from build123d import *

# Parameters (mm, degrees)
SKETCH1_W               = 100
SKETCH1_H               = 45
BOSS_EXTRUDE1_DEPTH     = 3
BOSS_EXTRUDE2_DEPTH     = 15
SKETCH4_R               = 1.5
CUT_EXTRUDE1_DEPTH      = 79
SKETCH5_R               = 1.5
CUT_EXTRUDE2_DEPTH      = 25
FILLET1_R               = 2
SKETCH6_W               = 3
SKETCH6_H               = 45
BOSS_EXTRUDE3_DEPTH     = 20
FILLET2_R               = 17
SKETCH7_R               = 1.75
CUT_EXTRUDE3_DEPTH      = 73.5
CIRPATTERN1_COUNT       = 5
CIRPATTERN1_ANGLE       = 80
MIRROR1_COPY_1_SKETCH_R = 1.75
MIRROR1_COPY_1_DEPTH    = 73.5
MIRROR1_COPY_2_SKETCH_R = 1.75
MIRROR1_COPY_2_DEPTH    = 73.5
MIRROR1_COPY_3_SKETCH_R = 1.75
MIRROR1_COPY_3_DEPTH    = 73.5
MIRROR1_COPY_4_SKETCH_R = 1.75
MIRROR1_COPY_4_DEPTH    = 73.5
SKETCH8_R               = 1.75
CUT_EXTRUDE4_DEPTH      = 24
LPATTERN1_COUNT         = 4
LPATTERN1_PITCH         = 5
MIRROR2_COPY_1_SKETCH_R = 1.75
MIRROR2_COPY_1_DEPTH    = 24
MIRROR2_COPY_2_SKETCH_R = 1.75
MIRROR2_COPY_2_DEPTH    = 24
MIRROR2_COPY_3_SKETCH_R = 1.75
MIRROR2_COPY_3_DEPTH    = 24


with BuildPart() as part:
    # Sketch1 → Boss-Extrude1 (new body)
    with BuildSketch(Plane(origin=(0, 0, 0), x_dir=(1, 0, 0), z_dir=(0, 1, 0))):
        Rectangle(SKETCH1_W, SKETCH1_H)
    extrude(amount=BOSS_EXTRUDE1_DEPTH)

    # Sketch2 → Boss-Extrude2 (add)
    with BuildSketch(Plane(origin=(0, 3, 0), x_dir=(1, 0, 0), z_dir=(0, 1, 0))):
        Polygon((-25, 22.5), (-28, 22.5), (-28, -22.5), (-25, -22.5), (-25, -1.5), (25, -1.5), (25, -22.5), (28, -22.5), (28, 22.5), (25, 22.5), (25, 1.5), (-25, 1.5), align=None)
    extrude(amount=BOSS_EXTRUDE2_DEPTH)

    # Sketch4 → Cut-Extrude1 (cut, through all)
    with BuildSketch(Plane.ZY.offset(28)):
        with Locations((-18.5, 9.88505799)):
            Circle(SKETCH4_R)
        with Locations((18.5, 9.88505799)):
            Circle(SKETCH4_R)
    extrude(amount=-CUT_EXTRUDE1_DEPTH, mode=Mode.SUBTRACT)

    # Sketch5 → Cut-Extrude2 (cut, through all)
    with BuildSketch(Plane.XY.offset(1.5)):
        with Locations((-18.5, 9.963459829)):
            Circle(SKETCH5_R)
        with Locations((18.5, 9.963459829)):
            Circle(SKETCH5_R)
    extrude(amount=-CUT_EXTRUDE2_DEPTH, mode=Mode.SUBTRACT)

    # Fillet1
    fillet1_edges = [part.edges().sort_by_distance(p)[0] for p in [
        (-26.5, 18, 22.5),
        (26.5, 18, 22.5),
        (26.5, 18, -22.5),
        (-26.5, 18, -22.5),
        (50, 1.5, 22.5),
        (-50, 1.5, 22.5),
        (-50, 1.5, -22.5),
        (50, 1.5, -22.5),
    ]]
    fillet(fillet1_edges, radius=FILLET1_R)

    # Sketch6 → Boss-Extrude3 (add)
    with BuildSketch(Plane.XZ):
        with Locations((-21, 0)):
            Rectangle(SKETCH6_W, SKETCH6_H)
        with Locations((21, 0)):
            Rectangle(SKETCH6_W, SKETCH6_H)
    extrude(amount=BOSS_EXTRUDE3_DEPTH)

    # Fillet2
    fillet2_edges = [part.edges().sort_by_distance(p)[0] for p in [
        (-21, -20, 22.5),
        (-21, -20, -22.5),
        (21, -20, -22.5),
        (21, -20, 22.5),
    ]]
    fillet(fillet2_edges, radius=FILLET2_R)

    # Sketch7 → Cut-Extrude3 (cut, through all)
    with BuildSketch(Plane(origin=(22.5, 0, 0), x_dir=(0, 0, -1), z_dir=(1, 0, 0))):
        with Locations((5.5, -17)):
            Circle(SKETCH7_R)
    cut_extrude3 = extrude(amount=-CUT_EXTRUDE3_DEPTH, mode=Mode.SUBTRACT)

    # CirPattern1: Cut-Extrude3 ×5 about axis
    cirpattern1_axis = Axis((0, -3, -5.5), (1, 0, 0))
    for i in range(1, CIRPATTERN1_COUNT):
        add(cut_extrude3.rotate(cirpattern1_axis, i * CIRPATTERN1_ANGLE / (CIRPATTERN1_COUNT - 1)), mode=Mode.SUBTRACT)

    # Mirror1: Cut-Extrude3 across plane
    add(cut_extrude3.mirror(Plane.XY), mode=Mode.SUBTRACT)

    # Mirror1 copy 1 sketch → Mirror1 copy 1 (cut, through all)
    with BuildSketch(Plane(origin=(22.5, -2.062032926, -0.694369844), x_dir=(0, 0.342020143, 0.939692621), z_dir=(1, 0, 0))):
        with Locations((5.5, 17)):
            Circle(MIRROR1_COPY_1_SKETCH_R)
    extrude(amount=-MIRROR1_COPY_1_DEPTH, mode=Mode.SUBTRACT)

    # Mirror1 copy 2 sketch → Mirror1 copy 2 (cut, through all)
    with BuildSketch(Plane(origin=(22.5, -4.237198524, -0.641607266), x_dir=(0, 0.64278761, 0.766044443), z_dir=(1, 0, 0))):
        with Locations((5.5, 17)):
            Circle(MIRROR1_COPY_2_SKETCH_R)
    extrude(amount=-MIRROR1_COPY_2_DEPTH, mode=Mode.SUBTRACT)

    # Mirror1 copy 3 sketch → Mirror1 copy 3 (cut, through all)
    with BuildSketch(Plane(origin=(22.5, -6.263139721, 0.151923789), x_dir=(0, 0.866025404, 0.5), z_dir=(1, 0, 0))):
        with Locations((5.5, 17)):
            Circle(MIRROR1_COPY_3_SKETCH_R)
    extrude(amount=-MIRROR1_COPY_3_DEPTH, mode=Mode.SUBTRACT)

    # Mirror1 copy 4 sketch → Mirror1 copy 4 (cut, through all)
    with BuildSketch(Plane(origin=(22.5, -7.895498109, 1.590511764), x_dir=(0, 0.984807753, 0.173648178), z_dir=(1, 0, 0))):
        with Locations((5.5, 17)):
            Circle(MIRROR1_COPY_4_SKETCH_R)
    extrude(amount=-MIRROR1_COPY_4_DEPTH, mode=Mode.SUBTRACT)

    # Sketch8 → Cut-Extrude4 (cut, through all)
    with BuildSketch(Plane(origin=(0, 3, 0), x_dir=(1, 0, 0), z_dir=(0, 1, 0))):
        with Locations((-15.5, 19.5)):
            Circle(SKETCH8_R)
        with Locations((15.5, 19.5)):
            Circle(SKETCH8_R)
    cut_extrude4 = extrude(amount=-CUT_EXTRUDE4_DEPTH, mode=Mode.SUBTRACT)

    # LPattern1: Cut-Extrude4 ×4
    with Locations(*[(0, 0, i * LPATTERN1_PITCH) for i in range(1, LPATTERN1_COUNT)]):
        add(cut_extrude4, mode=Mode.SUBTRACT)

    # Mirror2: Cut-Extrude4 across plane
    add(cut_extrude4.mirror(Plane.XY), mode=Mode.SUBTRACT)

    # Mirror2 copy 1 sketch → Mirror2 copy 1 (cut, through all)
    with BuildSketch(Plane(origin=(0, 3, -5), x_dir=(1, 0, 0), z_dir=(0, 1, 0))):
        with Locations((-15.5, -19.5)):
            Circle(MIRROR2_COPY_1_SKETCH_R)
        with Locations((15.5, -19.5)):
            Circle(MIRROR2_COPY_1_SKETCH_R)
    extrude(amount=-MIRROR2_COPY_1_DEPTH, mode=Mode.SUBTRACT)

    # Mirror2 copy 2 sketch → Mirror2 copy 2 (cut, through all)
    with BuildSketch(Plane(origin=(0, 3, -10), x_dir=(1, 0, 0), z_dir=(0, 1, 0))):
        with Locations((-15.5, -19.5)):
            Circle(MIRROR2_COPY_2_SKETCH_R)
        with Locations((15.5, -19.5)):
            Circle(MIRROR2_COPY_2_SKETCH_R)
    extrude(amount=-MIRROR2_COPY_2_DEPTH, mode=Mode.SUBTRACT)

    # Mirror2 copy 3 sketch → Mirror2 copy 3 (cut, through all)
    with BuildSketch(Plane(origin=(0, 3, -15), x_dir=(1, 0, 0), z_dir=(0, 1, 0))):
        with Locations((-15.5, -19.5)):
            Circle(MIRROR2_COPY_3_SKETCH_R)
        with Locations((15.5, -19.5)):
            Circle(MIRROR2_COPY_3_SKETCH_R)
    extrude(amount=-MIRROR2_COPY_3_DEPTH, mode=Mode.SUBTRACT)


solid = part.part
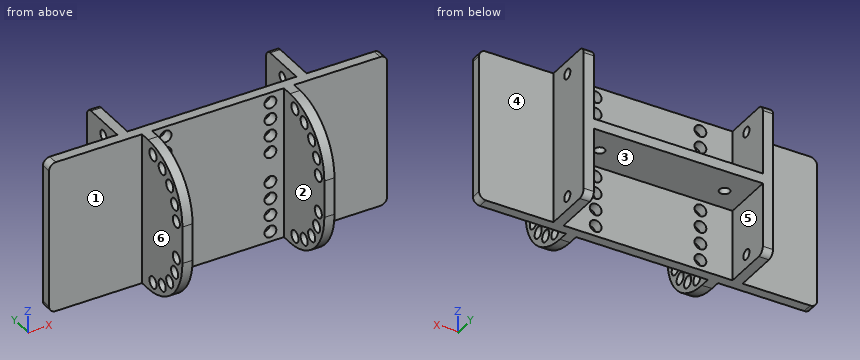
Work out the finished part from the listing and answer in its coordinate system (mm). Face numbers are marked on the shaded views. A direction names the side the tool comes from. Give positions to 0.01 mm unless a question says otherwise; leave off trailing zeros. Write each loop counter-clockwise with the first axis right and the second up, starting at its lowest first coordinate (ties: lowest second). Pieces come first, ordered by that corner, then holes. Notation, with made-up numbers: (66.25, -24.5) - (104.25, -24.5) arc R11 cw to (104.25, -4.5) - close; hole circle Ø2 at (78, 80). An arc over 180 degrees is marked (long way). One line per item, written item: value. Start each with the question number.
1. Consider probe 1 along Y at (x, z) = (27, -18.5); probe 2 along X at (y, z) = (9, 10); probe 3 along X at (y, z) = (0.75, 19.5). Determine where each line is inside the solid, lowest interval first.
2. Find section B-B (y = 6). Write down the section's boundary in (x, z).
3. Find section D-D (x = -4.5). Write down the section's boundary in (y, z), then the cut area to 3 significant figures.
4. Find section A-A (x = -18.5). Write down the section's boundary in (y, z).
5. Given pin 1 (4.5 mm diameter, centred on y = -10, z = -17.62, fed in from +X); pin 2 (5 mm diameter, centred on x = 40, z = -2.5, fed in from -Y); pin 3 (4.5 mm diameter, centred on x = -3.5, y = 7, fed in from -Z), each flat-ended and moving along its own axis, determine where each tip first touches the part or whether it passes through.
6. For a pull along X with two mould halves and no side action, classify the marked faces 4, 5 and 6 as +X half, -X half, draft (parallel to the pull), parting line (faces both ways), or undercut.
7. Find section C-C (x = 15.5). State how many separate pieces and enclosed holes the cut face has, then the cut area to 3 significant figures.
8. For the marked faces 1, 2 and 3, determine the directions among +Z, -Z, +X, -X, +Y, -Y from which every point of the face is accessible in a straight line to the end or side of a thin tool.
Geometry results:
1. probe 1: 0 to 8.39, 11.39 to 18
1. probe 2: -28 to -25, 25 to 28
1. probe 3: -50 to -17.25, -13.75 to 13.75, 17.25 to 50
2. outline: (-28, -22.5) - (-25, -22.5) - (-25, -1.5) - (25, -1.5) - (25, -22.5) - (28, -22.5) - (28, 22.5) - (25, 22.5) - (25, 1.5) - (-25, 1.5) - (-25, 22.5) - (-28, 22.5) - close
3. outline: (0, -22.5) - (3, -22.5) - (3, -1.5) - (18, -1.5) - (18, 1.5) - (3, 1.5) - (3, 22.5) - (0, 22.5) - close
3. area: 180 mm2
4. outline: (0, -22.5) - (3, -22.5) - (3, -1.5) - (8.46, -1.5) - (8.46, 1.5) - (3, 1.5) - (3, 22.5) - (0, 22.5) - close; (11.46, -1.5) - (18, -1.5) - (18, 1.5) - (11.46, 1.5) - close
5. pin 1: x = 22.5
5. pin 2: y = 0
5. pin 3: z = -1.5
6. face 4: draft
6. face 5: undercut
6. face 6: -X half
7. separate pieces: 9
7. enclosed holes: 0
7. area: 96.0 mm2
8. face 1: +Z, -Z, -X, -Y
8. face 2: +Z, -Z, -Y
8. face 3: -Z, +Y
